Can you work these out from the model? Positions are in its coordinate system, mm. A direction names the side the tool comes from. Give positions to 0.01 mm unless a question says otherwise; leave off trailing zeros. Loops run counter-clockwise (first coordinate to the right, second up) from the corner with the lowest first, then second, coordinate; pieces in that order, holes last. Notation, with made-up numbers: (52.25, -19) - (59.25, -19) arc R16 cw to (59.25, 3) - close; hole circle Ø11 at (-39, -22). An arc over 180 degrees is marked (long way). Answer in a Markdown table with one row per item.
from build123d import *

# Parameters (mm, degrees)
F1_DEPTH = 10
F2_R     = 3.25
F3_DEPTH = 25
F5_DEPTH = 3


with BuildPart() as f1:
    # F0 (on Front) → F1 (new body, symmetric)
    with BuildSketch(Plane.XZ):
        with BuildLine():
            Line((0, 3), (0, 0))
            Line((0, 0), (20.171573, 0))
            ThreePointArc((20.171573, 0), (22.019332, 1.234633), (21.585786, 3.414214))
            Line((21.585786, 3.414214), (10.857864, 14.142136))
            Line((10.857864, 14.142136), (3.786797, 7.071068))
            Line((3.786797, 7.071068), (4.443651, 6.414214))
            ThreePointArc((4.443651, 6.414214), (4.877196, 4.234633), (3.029437, 3))
            Line((3.029437, 3), (0, 3))
        make_face()
    extrude(amount=F1_DEPTH, both=True)

    # F2 (on face) → F3 (cut)
    with BuildSketch(Plane(origin=(-1.642136, 0, 1.642136), x_dir=(0, -1, 0), z_dir=(-0.707107, 0, 0.707107))):
        with Locations((-4, 12.67767)):
            Circle(F2_R)
        with Locations((4, 12.67767)):
            Circle(F2_R)
    extrude(amount=-F3_DEPTH, mode=Mode.SUBTRACT)

    # F4 (on Top) → F5 (join)
    with BuildSketch(Plane.XY):
        with BuildLine():
            Line((0, -10), (0, 10))
            Line((0, 10), (-58, 10))
            ThreePointArc((-58, 10), (-59.414214, 9.414214), (-60, 8))
            Line((-60, 8), (-60, -8))
            ThreePointArc((-60, -8), (-59.414214, -9.414214), (-58, -10))
            Line((-58, -10), (0, -10))
        make_face()
        with BuildLine():
            Line((-53, 6), (-7, 6))
            ThreePointArc((-7, 6), (-5.585786, 5.414214), (-5, 4))
            Line((-5, 4), (-5, -4))
            ThreePointArc((-5, -4), (-5.585786, -5.414214), (-7, -6))
            Line((-7, -6), (-53, -6))
            ThreePointArc((-53, -6), (-54.414214, -5.414214), (-55, -4))
            Line((-55, -4), (-55, 4))
            ThreePointArc((-55, 4), (-54.414214, 5.414214), (-53, 6))
        make_face(mode=Mode.SUBTRACT)
    extrude(amount=F5_DEPTH)


solid = f1.part
Q1. Imagine slicing it at B-B, the plane x = -51. Write out the boundary of the cut face in (y, z), and give its area (3 significant figures).
Checked values:
| item | result |
|---|---|
| outline | (-10, 0) - (-6, 0) - (-6, 3) - (-10, 3) - close; (6, 0) - (10, 0) - (10, 3) - (6, 3) - close |
| area | 24.0 mm² |
Q2. Imagine slicing it at C-C, the plane y = 3. Write out the boundary of the cut face in (x, z).
Checked values:
| item | result |
|---|---|
| outline | (-60, 0) - (-55, 0) - (-55, 3) - (-60, 3) - close; (-5, 0) - (13.56, 0) - (5.14, 8.42) - (3.79, 7.07) - (4.44, 6.41) arc R2 cw to (3.03, 3) - (-5, 3) - close; (9.51, 12.79) - (21.65, 0.65) arc R2 ccw to (21.59, 3.41) - (10.86, 14.14) - close |
Q3. Imagine slicing it at A-A, the plane y = -2.5. Write out the boundary of the cut face in (x, z).
Checked values:
| item | result |
|---|---|
| outline | (-60, 0) - (-55, 0) - (-55, 3) - (-60, 3) - close; (-5, 0) - (13.85, 0) - (5.28, 8.57) - (3.79, 7.07) - (4.44, 6.41) arc R2 cw to (3.03, 3) - (-5, 3) - close; (9.36, 12.65) - (21.5, 0.51) arc R2 ccw to (21.59, 3.41) - (10.86, 14.14) - close |
Q4. On a 3-axis mill with a long thin cutter (end or side, diameter ignored), from which of +Z, -Z, +X, -X, +Y, -Y can I reach the whole of each face in a straight line? I mean faces 1 (the face through (-60, 0, 1)), 2 (the face through (-54.4, -5.43, 1.48)). Say none if no direction works.
Checked values:
| item | result |
|---|---|
| face 1 | +Z, -Z, -X, +Y, -Y |
| face 2 | +Z, -Z |
Q5. Imagine slicing it at D-D, the plane x = -1.5. Write out the boundary of the cut face in (y, z), and give its area (3 significant figures).
Checked values:
| item | result |
|---|---|
| outline | (-10, 0) - (10, 0) - (10, 3) - (-10, 3) - close |
| area | 60.0 mm² |
Q6. If I drill on line 1 (Y direction, x = 10.5, z = 7.5); line 2 (Y direction, x = -41, z = 2.25); line 3 (X direction, y = -4.25, z = 2), over which ranges is the centre line in solid material (lowest first)? Write a range as [from, to].
Checked values:
| item | result |
|---|---|
| line 1 | y = [-10, -7.25], [-0.75, 0.75], [7.25, 10] |
| line 2 | y = [-10, -6], [6, 10] |
| line 3 | x = [-60, -54.98], [-5.02, 11.35], [20.51, 22.17] |
Q7. If we mould it in two halves opening along Y, with no side actions, what happens to faces 3 (the face through (14.24, 4.423, 8.246)), 4 (the face through (-59.43, -9.4, 1.48)), 5 (the face through (16, 0, 9))? For each: released by +Y, released by -Y, zero draft, split by the parting line, or undercut.
Checked values:
| item | result |
|---|---|
| face 3 | undercut |
| face 4 | released by -Y |
| face 5 | zero draft |
Q8. For pin 1 (12 mm diameter, centred on x = -42.5, y = -8, fed in from -Z), with a flat end and sliding along its axis, tell me the tip position at first contact or that it passes through.
Checked values:
| item | result |
|---|---|
| pin 1 | stops at z = 0 |
